```python
from build123d import *

# Parameters (mm, degrees)
BOSS_EXTRUDE1_DEPTH            = 86.5
M3X0_5_TAPPED_HOLE2_AT_2_COUNT = 2
M3X0_5_TAPPED_HOLE2_AT_2_PITCH = 23.4
M3X0_5_TAPPED_HOLE1_AT_2_COUNT = 2
M3X0_5_TAPPED_HOLE1_AT_2_PITCH = 46.8


with BuildPart() as part:
    # Sketch1 → Boss-Extrude1 (new body)
    with BuildSketch(Plane.XY):
        Polygon((0, 0), (0, 56.8), (8.5, 56.8), (8.5, 46.8), (2.5, 46.8), (2.5, 45.1), (8.5, 45.1), (8.5, 35.1), (2.5, 35.1), (2.5, 33.4), (8.5, 33.4), (8.5, 23.4), (2.5, 23.4), (2.5, 21.7), (8.5, 21.7), (8.5, 11.7), (2.5, 11.7), (2.5, 10), (8.5, 10), (8.5, 0), align=None)
    extrude(amount=BOSS_EXTRUDE1_DEPTH)

    # Sketch4 → M3x0.5 Tapped Hole2 (revolve, cut)
    with BuildSketch(Plane(origin=(4.25, 40.1, 86.5), x_dir=(0, -1, 0), z_dir=(1, 0, 0))):
        Polygon((0, 0), (0, 5.751075774), (1.25, 5), (1.25, 0), align=None)
    m3x0_5_tapped_hole2 = revolve(axis=Axis((4.25, 40.1, 92.85), (0, 0, -1)), mode=Mode.SUBTRACT)

    # M3x0.5 Tapped Hole2 at 2: M3x0.5 Tapped Hole2 ×2
    with Locations(*[(0, -i * M3X0_5_TAPPED_HOLE2_AT_2_PITCH, 0) for i in range(1, M3X0_5_TAPPED_HOLE2_AT_2_COUNT)]):
        add(m3x0_5_tapped_hole2, mode=Mode.SUBTRACT)

    # Mirror1: M3x0.5 Tapped Hole2 across plane
    add(m3x0_5_tapped_hole2.mirror(Plane.XY.offset(43.25)), mode=Mode.SUBTRACT)

    # Mirror1 copy 1 sketch → Mirror1 copy 1 (revolve, cut)
    with BuildSketch(Plane(origin=(4.25, 16.7, 0), x_dir=(0, -1, 0), z_dir=(1, 0, 0))):
        Polygon((0, 0), (0, -5.751075774), (1.25, -5), (1.25, 0), align=None)
    revolve(axis=Axis((4.25, 16.7, -6.35), (0, 0, -1)), mode=Mode.SUBTRACT)

    # Sketch11 → M3x0.5 Tapped Hole1 (revolve, cut)
    with BuildSketch(Plane(origin=(0, 5, 8.25), x_dir=(0, 0, 1), z_dir=(0, 1, 0))):
        Polygon((0, 0), (0, 4.751075774), (1.25, 4), (1.25, 0), align=None)
    m3x0_5_tapped_hole1 = revolve(axis=Axis((-6.35, 5, 8.25), (1, 0, 0)), mode=Mode.SUBTRACT)

    # M3x0.5 Tapped Hole1 at 2: M3x0.5 Tapped Hole1 ×2
    with Locations(*[(0, i * M3X0_5_TAPPED_HOLE1_AT_2_PITCH, 0) for i in range(1, M3X0_5_TAPPED_HOLE1_AT_2_COUNT)]):
        add(m3x0_5_tapped_hole1, mode=Mode.SUBTRACT)

    # Mirror2: M3x0.5 Tapped Hole1 across plane
    add(m3x0_5_tapped_hole1.mirror(Plane(origin=(0, 0, 43.25), x_dir=(1, 0, 0), z_dir=(0, 0, -1))), mode=Mode.SUBTRACT)

    # Mirror2 copy 1 sketch → Mirror2 copy 1 (revolve, cut)
    with BuildSketch(Plane(origin=(0, 51.8, 78.25), x_dir=(0, 0, -1), z_dir=(0, 1, 0))):
        Polygon((0, 0), (0, -4.751075774), (1.25, -4), (1.25, 0), align=None)
    revolve(axis=Axis((-6.35, 51.8, 78.25), (-1, 0, 0)), mode=Mode.SUBTRACT)


solid = part.part
```
The listing builds one solid part. Answer for the finished solid, in the listing's coordinates (mm). A direction names the side the tool comes from. Round coordinates to 2 decimals unless told otherwise and drop trailing zeros. Write each loop counter-clockwise with the first axis right and the second up, starting at its lowest first coordinate (ties: lowest second). Pieces come first, ordered by that corner, then holes. Notation, with made-up numbers: (4.25, 65.25) -> (41.25, 65.25) arc R32 cw to (41.25, 92.25) -> close; hole circle Ø1 at (74, 12.25). An arc over 180 degrees is marked (long way). Use CSV: the item, a comma, the result in double quotes. Start each with the question number.
(1) The mould has two halves that part along Z. Classify faces 1 (the face through (2.5, 34, 43)), 2 (the face through (4.621, 5.132, 78.422)), 3 (the face through (4, 29, 86.5)): released by +Z, released by -Z, zero draft, split by the parting line, or undercut.
(2) Which of the six approach directions +Z, -Z, +X, -X, +Y, -Y give full straight-line access (tool end or side, diameter ignored) to faces 4 (the face through (4.24, 40.32, 80.88)), 5 (the face through (4.2, 17.95, 2.46)), 6 (the face through (5, 45.1, 43))?
(3) Each of these flat-tipped pins is pushed along its axis until it touches: pin 1 (3 mm diameter, centred on x = 4.25, y = 16.7, fed in from +Z); pin 2 (1.5 mm diameter, centred on y = 51.8, z = 8.25, fed in from -X); pin 3 (2 mm diameter, centred on x = 4.25, y = 40.1, fed in from -Z); pin 4 (2 mm diameter, centred on y = 51.8, z = 78.25, fed in from -X). Where does it stop, or does it pass through?
(4) Consider L1, parallel to Y at x = 7.5, z = 6.5; L2, parallel to Z at x = 1.1, y = 51.8; L3, parallel to X at y = 40.1, z = 82.9. Determine where each line is inside the solid, lowest interval first. Write a range as from..to.
(5) Section A-A on z = 56.5 is taken. Give the vertices of the cut face in (x, y).
A:
1,face 1,"zero draft"
1,face 2,"undercut"
1,face 3,"released by +Z"
2,face 4,"+Z"
2,face 5,"-Z"
2,face 6,"+Z, -Z, +X"
3,pin 1,"stops at z = 86.5"
3,pin 2,"stops at x = 4.3"
3,pin 3,"stops at z = 5.15"
3,pin 4,"stops at x = 4.15"
4,L1,"y = 0..10, 11.7..21.7, 23.4..33.4, 35.1..45.1, 46.8..56.8"
4,L2,"z = 0..7, 9.5..77, 79.5..86.5"
4,L3,"x = 0..3, 5.5..8.5"
5,outline,"(0, 0) -> (8.5, 0) -> (8.5, 10) -> (2.5, 10) -> (2.5, 11.7) -> (8.5, 11.7) -> (8.5, 21.7) -> (2.5, 21.7) -> (2.5, 23.4) -> (8.5, 23.4) -> (8.5, 33.4) -> (2.5, 33.4) -> (2.5, 35.1) -> (8.5, 35.1) -> (8.5, 45.1) -> (2.5, 45.1) -> (2.5, 46.8) -> (8.5, 46.8) -> (8.5, 56.8) -> (0, 56.8) -> close"
